The drawing under review shows one solid part. Ordinate dimensions are in mm from its lowest x, y, z. A direction names the side the tool comes from. Coordinates: 2 decimals unless noted, no trailing zeros. Loops run counter-clockwise (first coordinate to the right, second up) from the corner with the lowest first, then second, coordinate; pieces in that order, holes last. Notation, with made-up numbers: M 85.25,7 L 89.25,7 A5 ccw 89.25,14 Z; hole C 22.25,14.5 d11. An arc over 180 degrees is marked long. Answer as a JSON object with one key per item and string values. Group by question number.
1. Insertion check: pin 1 (3.5 mm diameter, centred on x = 25.5, y = 37, fed in from -Z); pin 2 (2 mm diameter, centred on x = 21, z = 15.5, fed in from -Y); pin 3 (1.5 mm diameter, centred on y = 98.5, z = 25.5, fed in from +X). Each pin has a flat end and moves straight along its axis. Give the tip position at first contact, or say it passes through.
2. To check wall thickness, follow probe 1 along Y at (x, z) = (25, 10.5); probe 2 along Y at (x, z) = (4, 19.75); probe 3 along Y at (x, z) = (20.5, 5.75). State the ranges of each line that lie inside material, in increasing order.
3. Machinability: for the marked faces 1 and 2, which of the approach directions +Z, -Z, +X, -X, +Y, -Y give a long, thin tool a straight path to every point of the face, cutting with its end or side? Answer none if there is none.
4. Consider section B-B (x = 25). State the section outline as (y, z) points, then the cut area to 3 significant figures.
5. Consider section D-D (x = 37.5). State the section outline as (y, z) points, then the cut area to 3 significant figures.
6. Draft analysis for pull direction X (two halves, no side actions). For the marked faces 3, 4 and 5, state which applies: +X half, -X half, draft (parallel to the pull), parting line (faces both ways), or undercut.
7. Consider section C-C (y = 35). State the section outline as (x, z) points, then the cut area to 3 significant figures.
8. Consider section A-A (z = 13.75). State the section outline as (x, y) points.
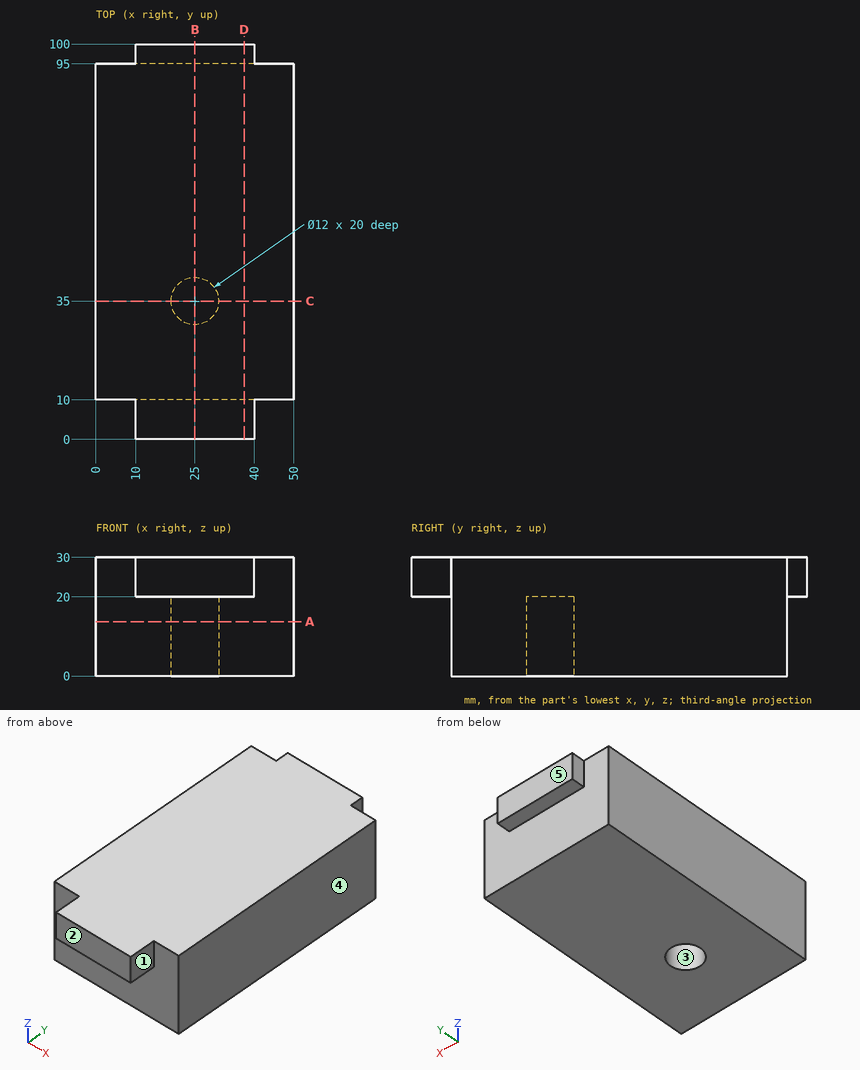
Findings below:
{
 "1": {"pin 1": "stops at z = 20", "pin 2": "stops at y = 10", "pin 3": "stops at x = 40"},
 "2": {"probe 1": "y = 10 to 29, 41 to 95", "probe 2": "y = 10 to 95", "probe 3": "y = 10 to 31.03, 38.97 to 95"},
 "3": {"face 1": "+Z, -Z, +X, -Y", "face 2": "+Z, -Z, +X, -X, -Y"},
 "4": {"outline": "M 0,20 L 10,20 L 10,0 L 29,0 L 29,20 L 41,20 L 41,0 L 95,0 L 95,20 L 100,20 L 100,30 L 0,30 Z", "area": "2,460 mm^2"},
 "5": {"outline": "M 0,20 L 10,20 L 10,0 L 95,0 L 95,20 L 100,20 L 100,30 L 0,30 Z", "area": "2,700 mm^2"},
 "6": {"face 3": "undercut", "face 4": "+X half", "face 5": "draft"},
 "7": {"outline": "M 0,0 L 19,0 L 19,20 L 31,20 L 31,0 L 50,0 L 50,30 L 0,30 Z", "area": "1,260 mm^2"},
 "8": {"outline": "M 0,10 L 50,10 L 50,95 L 0,95 Z; hole C 25,35 d12"}
}
